```python
from build123d import *

# Parameters (mm, degrees)
SKETCH_1_R      = 8
EXTRUDE_1_DEPTH = 10


with BuildPart() as part:
    # 草图1 → 凸台-拉伸1 (new body)
    with BuildSketch(Plane.XY):
        with BuildLine():
            ThreePointArc((-2.313590971, 15.831844391), (-16, 0), (-2.313590971, -15.831844391))
            add(Edge.make_bspline(
                [(-2.313590971, -15.831844391), (61.84269778, -25.207341442), (219.572103506, -39.191033108), (399.013095208, -23.620927123), (452.313590971, -15.831844391)],
                knots=[0, 0, 0, 0, 0.5, 1, 1, 1, 1], degree=3))
            ThreePointArc((452.313590971, -15.831844391), (466, 0), (452.313590971, 15.831844391))
            add(Edge.make_bspline(
                [(-2.313590971, 15.831844391), (61.84269778, 25.207341442), (219.572103506, 39.191033108), (399.013095208, 23.620927123), (452.313590971, 15.831844391)],
                knots=[0, 0, 0, 0, 0.5, 1, 1, 1, 1], degree=3))
        make_face()
        Circle(SKETCH_1_R, mode=Mode.SUBTRACT)
        with Locations((450, 0)):
            Circle(SKETCH_1_R, mode=Mode.SUBTRACT)
    extrude(amount=EXTRUDE_1_DEPTH)


solid = part.part
```
For this review, take the finished solid that the model builds, in its own axes (mm). Round coordinates to 2 decimals unless told otherwise and drop trailing zeros. Loops run counter-clockwise (first coordinate to the right, second up) from the corner with the lowest first, then second, coordinate; pieces in that order, holes last.
(1) We need section A-A (y = 0). Give the boundary of the cut face in (x, z).
Returned:
outline: (-16, 0) - (-8, 0) - (-8, 10) - (-16, 10) - close; (8, 0) - (442, 0) - (442, 10) - (8, 10) - close; (458, 0) - (466, 0) - (466, 10) - (458, 10) - close
(2) Mouldability with a two-part tool opening along Y and no side actions: class faces 1 (the flat face through (222, 1, 10)), 2 (the cylindrical face through (-1.73, -7.81, 4.93)), 3 (the cylindrical face through (-16, 0, 5)) as released by +Y, released by -Y, zero draft, split by the parting line, or undercut.
Returned:
face 1: zero draft
face 2: undercut
face 3: split by the parting line
(3) Clearance check with flat-ended pins moving along their axes: P1, Ø13, axis at x = 0, y = 0, coming from the +Z side; P2, Ø3, axis at y = -9.5, z = 1, coming from the +X side. State where each tip first meets the part, or that it passes through.
Returned:
P1: passes through
P2: stops at x = 463.86
(4) Wall thickness on line 1 along X through (y, z) = (-1, 1); line 2 along X through (y, z) = (4, 6.5); line 3 along Y through (x, z) = (450, 3.75): over which ranges is each line inside the solid? List them lowest first.
Returned:
line 1: x = -15.97 to -7.94, 7.94 to 442.06, 457.94 to 465.97
line 2: x = -15.49 to -6.93, 6.93 to 443.07, 456.93 to 465.49
line 3: y = -16.17 to -8, 8 to 16.17
(5) We need section B-B (z = 6). State how many separate pieces and enclosed holes the cut face has, plus the area to 3 significant figures.
Returned:
separate pieces: 1
enclosed holes: 2
area: 24,300 mm2
